from build123d import *

# Parameters (mm, degrees)
F0_W     = 30
F0_H     = 30
F0_W_2   = 13
F0_H_2   = 13
F0_R     = 1.9
F1_DEPTH = 5
F2_R     = 3.3
F2_R_2   = 1.7
F3_DEPTH = 3
F3_TAPER = 10
F4_W     = 30
F4_H     = 30
F5_DEPTH = 1
F6_R     = 0.5


with BuildPart() as f1:
    # F0 (on Top) → F1 (new body)
    with BuildSketch(Plane.XY):
        Rectangle(F0_W, F0_H)
        with Locations((-7.2, -7)):
            Rectangle(F0_W_2, F0_H_2, mode=Mode.SUBTRACT)
        with Locations((7.2, -7)):
            Rectangle(F0_W_2, F0_H_2, mode=Mode.SUBTRACT)
        with Locations((0, 3.4)):
            Circle(F0_R, mode=Mode.SUBTRACT)
    extrude(amount=F1_DEPTH)

    # F2 (on face) → F3 (join)
    with BuildSketch(Plane.XY.offset(5)):
        with Locations((0, 3.4)):
            Circle(F2_R)
        with Locations((0, 3.4)):
            Circle(F2_R_2, mode=Mode.SUBTRACT)
    extrude(amount=F3_DEPTH, taper=F3_TAPER)

    # F4 (on face) → F5 (join)
    with BuildSketch(Plane(origin=(0, 0, 0), x_dir=(1, 0, 0), z_dir=(0, 0, -1))):
        Rectangle(F4_W, F4_H)
    extrude(amount=F5_DEPTH)

    # F6
    f6_edges = [f1.edges().sort_by_distance(p)[0] for p in [
        (-15, -15, 2),
        (15, -15, 2),
        (15, 15, 2),
        (-15, 15, 2),
        (-3.3, 3.4, 5),
    ]]
    fillet(f6_edges, radius=F6_R)


solid = f1.part
Here's how the part is built. I have some questions about the finished solid (model axes, mm). A direction names the side the tool comes from. Give positions to 0.01 mm unless a question says otherwise; leave off trailing zeros. Write each loop counter-clockwise with the first axis right and the second up, starting at its lowest first coordinate (ties: lowest second). Pieces come first, ordered by that corner, then holes. Notation, with made-up numbers: (-16.75, 7) -> (2.25, 7) arc R12 cw to (2.25, 30) -> close; hole circle Ø7 at (-28.5, -30). An arc over 180 degrees is marked (long way). Use one line per item in the form item = value. Start each with the question number.
1. Imagine slicing it at B-B on y = -1.75. List the corners of the cut face in (x, z) for me.
2. Will these pins go through, and if not, where does the flat tip stop? pin 1 Ø4 at (x, y) = (8, -8.5) entering from +Z; pin 2 Ø5 at (x, y) = (7, -12) entering from +Z.
3. Imagine slicing it at D-D on x = 4.5. List the corners of the cut face in (y, z) for me, plus the area to 3 significant figures.
4. Thinking about a two-plate mould opening in Z: for faces 1 (the face through (0, 3, 0)), 2 (the face through (-2, 5, 8)), 3 (the face through (7, -0.5, 2)), which applies, +Z half, -Z half, draft (parallel to the pull), parting line (faces both ways), or undercut?
5. Imagine slicing it at C-C on x = 0. List the corners of the cut face in (y, z) for me.
6. If I drill on L1, parallel to X at y = -4.75, z = 2.5; L2, parallel to Y at x = -5.5, z = 2; L3, parallel to Y at x = 0, z = 3.5, over which ranges is the centre line in solid material (lowest first)?
7. On a 3-axis mill with a long thin cutter (end or side, diameter ignored), from which of +Z, -Z, +X, -X, +Y, -Y can I reach the whole of each face in a straight line? I mean faces 4 (the face through (-0.7, -7, 2)), 5 (the face through (15, 0, 2)). Say none if no direction works.
8. Imagine slicing it at A-A on z = 4.5. List the corners of the cut face in (x, y) for me.
Entries:
q1.outline = (-15, -1) -> (15, -1) -> (15, 5) -> (13.7, 5) -> (13.7, 0) -> (0.7, 0) -> (0.7, 5) -> (-0.7, 5) -> (-0.7, 0) -> (-13.7, 0) -> (-13.7, 5) -> (-15, 5) -> close
q2.pin_1 = 0
q2.pin_2 = 5
q3.outline = (-15, -1) -> (15, -1) -> (15, 5) -> (-0.5, 5) -> (-0.5, 0) -> (-13.5, 0) -> (-13.5, 5) -> (-15, 5) -> close
q3.area = 115 mm²
q4.face_1 = undercut
q4.face_2 = +Z half
q4.face_3 = draft
q5.outline = (-15, -1) -> (15, -1) -> (15, 5) -> (7.12, 5) arc R0.5 cw to (6.63, 5.41) -> (6.17, 8) -> (5.63, 8) -> (5.1, 5) -> (5.3, 5) -> (5.3, 0) -> (1.5, 0) -> (1.5, 5) -> (1.7, 5) -> (1.17, 8) -> (0.63, 8) -> (0.17, 5.41) arc R0.5 cw to (-0.32, 5) -> (-15, 5) -> close
q6.L1 = -15 to -13.7, -0.7 to 0.7, 13.7 to 15
q6.L2 = -15 to -13.5, -0.5 to 15
q6.L3 = -15 to 1.5, 5.3 to 15
q7.face_4 = +Z
q7.face_5 = +Z, -Z, +X, +Y, -Y
q8.outline = (-15, -14.5) arc R0.5 ccw to (-14.5, -15) -> (14.5, -15) arc R0.5 ccw to (15, -14.5) -> (15, 14.5) arc R0.5 ccw to (14.5, 15) -> (-14.5, 15) arc R0.5 ccw to (-15, 14.5) -> close; hole (-13.7, -13.5) -> (-0.7, -13.5) -> (-0.7, -0.5) -> (-13.7, -0.5) -> close; hole circle Ø3.8 at (0, 3.4); hole (0.7, -13.5) -> (13.7, -13.5) -> (13.7, -0.5) -> (0.7, -0.5) -> close
